Autodesk Inventor part; units mm, degrees
ref_plane "YZ Plane" through (0, 0, 0) normal (1, 0, 0) x (0, 1, 0)
ref_plane "XZ Plane" through (0, 0, 0) normal (0, 1, 0) x (-1, 0, 0)
ref_plane "XY Plane" through (0, 0, 0) normal (0, 0, 1) x (1, 0, 0)
sketch "Sketch1" plane through (0, 0, 0) normal (0, 1, 0) x (-1, 0, 0)
  arc A0 (-51.5269, -6.9638) -> (-48.7189, -4.3924) centre (-51.6928, -3.9638) ccw
  line L0 (-51.5269, -6.9638) -> (-53.0277, -6.9638)
  arc A1 (-53.0277, -6.9638) -> (-55.8647, -7.8466) centre (-53.0278, -11.9638) ccw
  arc A2 (-48.0059, -0.3912) -> (-48.7189, -2.9645) centre (-43.7189, -2.9645) ccw
  line L1 (-48.7189, -2.9645) -> (-48.7189, -4.3924)
  arc A3 (-44.3192, 1.9993) -> (-48.0059, -0.3912) centre (-43.7189, -2.9645) ccw
  arc A4 (-55.8647, -7.8466) -> (-57.9428, -11.046) centre (-53.0278, -11.9639) ccw
  arc A5 (-7.9592, -0.1638) -> (-12.0937, 1.9993) centre (-12.0765, -3.0006) ccw
  arc A6 (-7.0769, -2.9368) -> (-7.9592, -0.1638) centre (-12.0765, -3.0006) ccw
  arc A7 (-7.0717, -4.4481) -> (-4.4894, -7.4079) centre (-4.0718, -4.4371) ccw
  line L2 (-7.0717, -4.4481) -> (-7.0769, -2.9368)
  arc A8 (-0.4247, -8.1232) -> (-3.0701, -7.403) centre (-3.0107, -12.4029) ccw
  line L3 (-3.0701, -7.403) -> (-4.4894, -7.4079)
  arc A9 (2.1302, -12.0566) -> (-0.4247, -8.1232) centre (-2.8554, -12.4986) ccw
  line L4 (2.1302, -12.0566) -> (2.1302, -17.0566)
  line L5 (-57.9428, -11.046) -> (-57.9439, -17.046)
  line L6 (-57.9439, -17.046) -> (2.1302, -17.0566)
  line L7 (-44.3192, 1.9993) -> (-12.0937, 1.9993)
  arc A10 (-6.0769, -2.9289) -> (-7.1357, 0.4036) centre (-12.0765, -3.0006) ccw
  arc A11 (-7.1357, 0.4036) -> (-12.0953, 2.9993) centre (-12.0765, -3.0006) ccw
  line L8 (-12.0953, 2.9993) -> (-44.3767, 2.9993)
  arc A12 (-44.3767, 2.9993) -> (-48.8633, 0.1235) centre (-43.7189, -2.9645) ccw
  arc A13 (-48.8633, 0.1235) -> (-49.7189, -2.9645) centre (-43.7189, -2.9645) ccw
  line L9 (-49.7189, -2.9645) -> (-49.7189, -4.3135)
  arc A14 (-51.5573, -5.9638) -> (-49.7189, -4.3135) centre (-51.6928, -3.9638) ccw
  line L10 (-51.5573, -5.9638) -> (-53.0277, -5.9638)
  arc A15 (-53.0277, -5.9638) -> (-56.4321, -7.0231) centre (-53.0278, -11.9638) ccw
  arc A16 (-56.4321, -7.0231) -> (-58.9428, -10.9576) centre (-53.0278, -11.9639) ccw
  line L11 (-58.9428, -10.9576) -> (-58.9441, -18.0408)
  line L12 (3.1302, -18.0204) -> (3.1302, -12.0144)
  arc A17 (3.1302, -12.0144) -> (0.0768, -7.258) centre (-2.8554, -12.4986) ccw
  arc A18 (0.0768, -7.258) -> (-3.0776, -6.403) centre (-3.0107, -12.4029) ccw
  line L13 (-3.0776, -6.403) -> (-4.4139, -6.4076)
  arc A19 (-6.0717, -4.4446) -> (-4.4139, -6.4076) centre (-4.0718, -4.4371) ccw
  line L14 (-6.0717, -4.4446) -> (-6.0769, -2.9289)
  arc A20 (-4.577, -2.9177) -> (-5.9005, 1.2546) centre (-12.0765, -3.0006) ccw
  arc A21 (-5.9005, 1.2546) -> (-12.0976, 4.4993) centre (-12.0765, -3.0006) ccw
  line L15 (-12.0976, 4.4993) -> (-44.4545, 4.4993)
  arc A22 (-44.4545, 4.4993) -> (-50.1493, 0.8955) centre (-43.7189, -2.9645) ccw
  arc A23 (-50.1493, 0.8955) -> (-51.2189, -2.9645) centre (-43.7189, -2.9645) ccw
  line L16 (-51.2189, -2.9645) -> (-51.2189, -4.1372)
  arc A24 (-51.6249, -4.4638) -> (-51.2189, -4.1372) centre (-51.6928, -3.9638) ccw
  line L17 (-51.6249, -4.4638) -> (-53.0277, -4.4638)
  arc A25 (-53.0277, -4.4638) -> (-57.2832, -5.7879) centre (-53.0278, -11.9638) ccw
  arc A26 (-57.2832, -5.7879) -> (-60.4428, -10.8378) centre (-53.0278, -11.9639) ccw
  line L18 (-60.4428, -10.8378) -> (-60.4443, -19.5405)
  line L19 (4.6302, -19.5486) -> (4.6302, -11.9572)
  arc A27 (4.6302, -11.9572) -> (0.8291, -5.9601) centre (-2.8554, -12.4986) ccw
  arc A28 (0.8291, -5.9601) -> (-3.0882, -4.903) centre (-3.0107, -12.4029) ccw
  line L20 (-3.0882, -4.903) -> (-4.2426, -4.907)
  arc A29 (-4.5718, -4.4391) -> (-4.2426, -4.907) centre (-4.0718, -4.4371) ccw
  line L21 (-4.5718, -4.4391) -> (-4.577, -2.9177)
  line L22 (3.1302, -18.0204) -> (3.1302, -19.5486)
  line L23 (3.1302, -18.0204) -> (4.6584, -18.0204) construction
  line L24 (3.1302, -19.5486) -> (4.6302, -19.5486)
  line L25 (-58.9441, -18.0408) -> (-58.9441, -19.5405)
  line L26 (-58.9441, -19.5405) -> (-60.4443, -19.5405)
  line L27 (-58.9441, -19.5405) -> (-57.9439, -19.5405)
  line L28 (-57.9439, -19.5405) -> (-57.9439, -17.046)
  line L29 (3.1302, -19.5486) -> (2.1302, -19.5486)
  line L30 (2.1302, -19.5486) -> (2.1302, -17.0566)
  point P0 (0, 0)
  point P1 (0, 0)
  dimension "d5" = 5
  dimension "d6" = 6
  dimension "d8" = 3
  dimension "d11" = 1
  dimension "d12" = 1.5
  dimension "d13" = 90
  dimension "d16" = 1
extrude "Extrusion2" add sketch "Sketch1" along normal blind 10 contours L0 A1 A4 L5 L28 L27 L25 L11 A16 A15 L10 A14 L9 A13 A12 L8 A11 A10 L14 A19 L13 A18 A17 L12 L22 L29 L30 L4 A9 A8 L3 A7 L2 A6 A5 L7 A3 A2 L1 A0 | L26 L18 A26 A25 L17 A24 L16 A23 A22 L15 A21 A20 L21 A29 L20 A28 A27 L19 L24 L22 L12 A17 A18 L13 A19 L14 A10 A11 L8 A12 A13 L9 A14 L10 A15 A16 L11 L25
sketch "Sketch2" plane through (-2.1302, 0, -12.0566) normal (1, 0, 0) x (0, 0, -1)
  line L0 (7.492, 0) -> (7.492, 10)
  line L1 (7.492, 5) -> (5.492, 5)
  arc A0 (6.992, 5) -> (3.992, 5) centre (5.492, 5) ccw
  line L2 (5.492, 5) -> (3.992, 5)
  point P0 (-12.0566, 0)
  dimension "d19" = 2
  dimension "d21" = 1.5
revolve "Revolution1" add sketch "Sketch2" angle 360 about axis through (-2.1302, 5, -19.5486) along (0, 0, 1)
sketch "Sketch3" plane through (57.9439, 0, -19.5405) normal (-1, 0, 0) x (0, 0, 1)
  line L0 (0, 0) -> (0, 10)
  line L1 (0, 5) -> (2, 5)
  arc A0 (3.5, 5) -> (0.5, 5) centre (2, 5) ccw
  line L2 (2, 5) -> (3.5, 5)
  point P0 (19.5405, 0)
  point P1 (2, 5)
  dimension "d23" = 2
  dimension "d24" = 1.5
revolve "Revolution2" add sketch "Sketch3" angle 360 about axis through (57.9439, 5, -19.5405) along (0, 0, 1)
properties part number "NEMA23_Shroud_Cover"
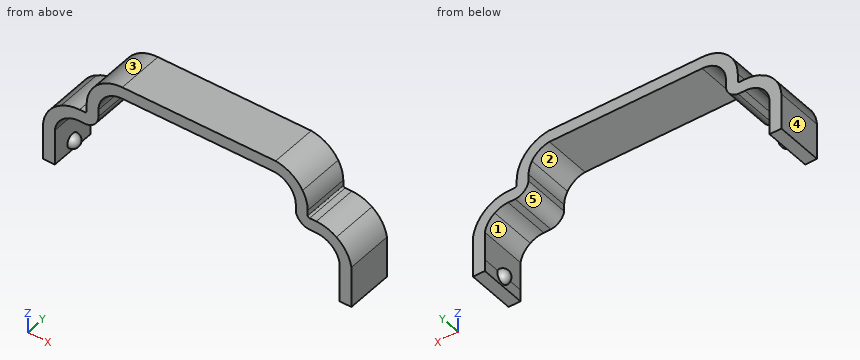
Geometry check sheet. Reference: the model listing, model coordinates, mm. Face numbers are marked on the shaded views. A direction names the side the tool comes from. Give positions to 0.01 mm unless a question says otherwise; leave off trailing zeros. Write each loop counter-clockwise with the first axis right and the second up, starting at its lowest first coordinate (ties: lowest second). Pieces come first, ordered by that corner, then holes.
1) Cross-section at D-D (x = 46). Record the boundary of the cut face in (y, z).
Values follow:
outline: (0, 1.48) - (10, 1.48) - (10, 4.18) - (0, 4.18) - close
2) Go/stop test with flat-tipped pins: pin 1 Ø0.8 at (x, y) = (60, 3) entering from -Z; pin 2 Ø1 at (x, y) = (35.5, 6.5) entering from -Z; pin 3 Ø1.6 at (y, z) = (2.5, -4) entering from -X; pin 4 Ø12 at (x, z) = (30, -4.5) entering from -Y. Record where each tip stops, or that it passes through.
Values follow:
pin 1: stops at z = -19.54
pin 2: stops at z = 2
pin 3: stops at x = 4.42
pin 4: passes through
3) Cross-section at A-A (z = -1.75). Record the boundary of the cut face in (x, y).
Values follow:
outline: (4.68, 0) - (7.24, 0) - (7.24, 10) - (4.68, 10) - close; (48.57, 0) - (51.12, 0) - (51.12, 10) - (48.57, 10) - close
4) Cross-section at B-B (x = 23.5). Record the boundary of the cut face in (y, z).
Values follow:
outline: (0, 2) - (10, 2) - (10, 4.5) - (0, 4.5) - close
5) Release check for a two-part mould opening along Z. For the marked faces 1, 2 and 3 record: released by +Z, released by -Z, zero draft, split by the parting line, or undercut.
Values follow:
face 1: undercut
face 2: released by -Z
face 3: released by +Z
6) Thickness scan on line 1 (X direction, y = 4, z = -16); line 2 (X direction, y = 3.5, z = -4); line 3 (Z direction, x = 28.5, y = 6.25). Record the ranges inside material, lowest first.
Values follow:
line 1: x = -4.63 to -2.13, 57.94 to 60.44
line 2: x = 4.57 to 7.07, 48.72 to 51.22
line 3: z = 2 to 4.5
7) Set-up check for the marked faces 4 and 5: record each of +Z, -Z, +X, -X, +Y, -Y from which the full face is reachable in a straight line by a thin tool's end or side.
Values follow:
face 4: +Z, -Z, -X, +Y, -Y
face 5: -Z, +Y, -Y
8) Cross-section at C-C (z = -9). Record the boundary of the cut face in (x, y).
Values follow:
outline: (-3.78, 0) - (-0.72, 0) - (-0.72, 10) - (-3.78, 10) - close; (57.05, 0) - (59.92, 0) - (59.92, 10) - (57.05, 10) - close
